Can you work these out from the drawing? Everything is in mm from the part's minimum corner. Round coordinates to 2 decimals unless told otherwise and drop trailing zeros. Loops run counter-clockwise (first coordinate to the right, second up) from the corner with the lowest first, then second, coordinate; pieces in that order, holes last. Notation, with made-up numbers: M -13.5,-31.75 L 4.5,-31.75 A21 ccw 4.5,-6.75 Z; hole C 63,69 d10. An arc over 180 degrees is marked long. One line per question, with ' | ' between items. Start each with the question number.
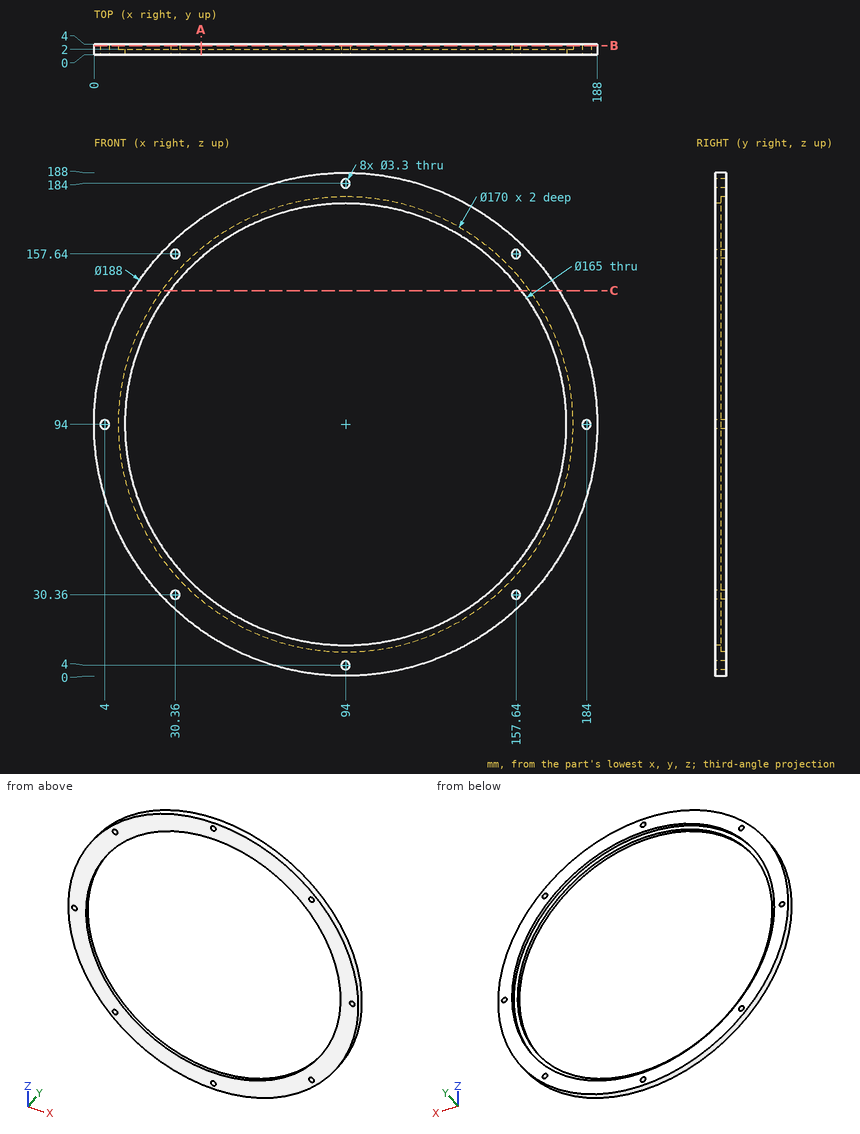
1) I'm going to push flat-ended pins straight in: pin 1 Ø2 at (x, z) = (94, 184) entering from +Y; pin 2 Ø1 at (y, z) = (1.5, 160.5) entering from -X; pin 3 Ø2 at (y, z) = (3, 127) entering from +X (1 decimal); pin 4 Ø1 at (x, y) = (151, 0.5) entering from -Z (1 decimal). Where does each tip first touch, or does it pass through?
2) Imagine slicing it at A-A (x = 40). Write out the boundary of the cut face in (y, z).
3) Imagine slicing it at C-C (z = 144). Write out the boundary of the cut face in (x, y).
4) Imagine slicing it at B-B (y = 3.35). State how many separate pieces and enclosed holes the cut face has, then the cut area to 3 significant figures.
5) Please list where these lines run through material, in increasing order: L1, parallel to Z at x = 94, y = 2.5; L2, parallel to Z at x = 29, y = 2.9 (1 decimal); L3, parallel to X at y = 1.35, z = 159 (1 decimal). Write a range as from..to.
Results are:
1) pin 1: through | pin 2: x = 27.07 | pin 3: x = 182.4 | pin 4: z = 18.9
2) outline: M 0,17.06 L 4,17.06 L 4,28.36 L 2,28.36 L 2,31.63 L 0,31.63 Z; M 0,156.37 L 2,156.37 L 2,159.64 L 4,159.64 L 4,170.94 L 0,170.94 Z
3) outline: M 14.4,0 L 28.38,0 L 28.38,2 L 25.26,2 L 25.26,4 L 14.4,4 Z; M 159.62,0 L 173.6,0 L 173.6,4 L 162.74,4 L 162.74,2 L 159.62,2 Z
4) separate pieces: 1 | enclosed holes: 9 | area: 4,990 mm²
5) L1: 0..2.35, 5.65..9, 179..182.35, 185.65..188 | L2: 26.1..29.4, 31.3..39.2, 148.8..156.7, 158.6..161.9 | L3: 26.1..29.4, 31.3..43.2, 144.8..156.7, 158.6..161.9
